```python
from build123d import *

# Parameters (mm, degrees)
F0_W     = 76.127068
F0_H     = 45.85968
F1_DEPTH = 2
F3_DEPTH = 2.001


with BuildPart() as f1:
    # F0 (on Front) → F1 (new body)
    with BuildSketch(Plane.XZ):
        Rectangle(F0_W, F0_H)
    extrude(amount=F1_DEPTH)

    # F2 (on face) → F3 (cut, through all)
    with BuildSketch(Plane.XZ.offset(2)):
        with BuildLine():
            Line((-22.34818, -8.622167), (-21.188844, -8.622167))
            Line((-21.188844, -8.622167), (-21.188844, 8.622167))
            ThreePointArc((-21.188844, 8.622167), (-20.0769, 9.734111), (-18.964956, 8.622167))
            Line((-18.964956, 8.622167), (-18.964956, -8.622167))
            ThreePointArc((-18.964956, -8.622167), (-17.090918, -10.496205), (-15.21688, -8.622167))
            Line((-15.21688, -8.622167), (-15.21688, 8.622167))
            Line((-15.21688, 8.622167), (-16.059408, 8.622167))
            Line((-16.059408, 8.622167), (-16.059408, -8.622167))
            ThreePointArc((-16.059408, -8.622167), (-16.852695, -9.415454), (-17.645983, -8.622167))
            Line((-17.645983, -8.622167), (-17.645983, 8.622167))
            ThreePointArc((-17.645983, 8.622167), (-19.997082, 10.973265), (-22.34818, 8.622167))
            Line((-22.34818, 8.622167), (-22.34818, -8.622167))
        make_face()
    extrude(amount=-F3_DEPTH, mode=Mode.SUBTRACT)


solid = f1.part
```
Input: part model. Units: mm. Frame: model coordinates. A direction names the side the tool comes from. Round coordinates to 2 decimals unless told otherwise and drop trailing zeros. Loops run counter-clockwise (first coordinate to the right, second up) from the corner with the lowest first, then second, coordinate; pieces in that order, holes last. Notation, with made-up numbers: M -3.5,65 L 32.5,65 A10 cw 32.5,70 Z; hole C 47.5,33.5 d5. An arc over 180 degrees is marked long. Answer in a Markdown table with one row per item. Add a question column.
1. Set-up query: faces 5 (the face through (-16.835, -1.014, -9.415)), 6 (the face through (-38.064, -1, 0)). Return all of +Z, -Z, +X, -X, +Y, -Y with unobstructed straight access to the full face (end or side cutting, diameter ignored); none if empty.
2. Section B-B (y = -0.7). Output: boundary loops of the cut face in (x, z).
3. Ray query, probe 1 along X at (y, z) = (-0.5, 0); probe 2 along X at (y, z) = (-0.6, 9); probe 3 along Z at (x, y) = (-22, -0.3). Return the intervals inside material, ascending.
4. Mould query, pull axis Z, two halves, no side actions, for faces 1 (the face through (-1, -1, -22.93)), 2 (the face through (-1, -1, 22.93)), 3 (the face through (-1, -2, 0)), 4 (the face through (-15.217, -1, 0)). Classes: released by +Z, released by -Z, zero draft, split by the parting line, or undercut.
5. Section A-A (z = -3.5). Output: boundary loops of the cut face in (x, y), and give its area (3 significant figures).
Values follow:
| question | item | result |
|---|---|---|
| 1 | face 5 | +Y, -Y |
| 1 | face 6 | +Z, -Z, -X, +Y, -Y |
| 2 | outline | M -38.06,-22.93 L 38.06,-22.93 L 38.06,22.93 L -38.06,22.93 Z; hole M -22.35,-8.62 L -21.19,-8.62 L -21.19,8.62 A1.11 cw -18.96,8.62 L -18.96,-8.62 A1.87 ccw -15.22,-8.62 L -15.22,8.62 L -16.06,8.62 L -16.06,-8.62 A0.79 cw -17.65,-8.62 L -17.65,8.62 A2.35 ccw -22.35,8.62 Z |
| 3 | probe 1 | -38.06 to -22.35, -21.19 to -18.96, -17.65 to -16.06, -15.22 to 38.06 |
| 3 | probe 2 | -38.06 to -22.32, -21.12 to -19.03, -17.68 to 38.06 |
| 3 | probe 3 | -22.93 to -8.62, 9.85 to 22.93 |
| 4 | face 1 | released by -Z |
| 4 | face 2 | released by +Z |
| 4 | face 3 | zero draft |
| 4 | face 4 | undercut |
| 5 | outline | M -38.06,-2 L -22.35,-2 L -22.35,0 L -38.06,0 Z; M -21.19,-2 L -18.96,-2 L -18.96,0 L -21.19,0 Z; M -17.65,-2 L -16.06,-2 L -16.06,0 L -17.65,0 Z; M -15.22,-2 L 38.06,-2 L 38.06,0 L -15.22,0 Z |
| 5 | area | 146 mm^2 |
